```python
from build123d import *

# Parameters (mm, degrees)
BOSS_EXTRUDE1_DEPTH = 20
SKETCH2_R           = 10
BOSS_EXTRUDE2_DEPTH = 150
SKETCH3_R           = 6
CUT_EXTRUDE1_DEPTH  = 197.643421463


with BuildPart() as part:
    # Sketch1 → Boss-Extrude1 (new body)
    with BuildSketch(Plane.XY):
        with BuildLine():
            Line((-3.960100717, 69.887893103), (-2.25, 65.189429999))
            Line((-2.25, 65.189429999), (2.25, 65.189429999))
            Line((2.25, 65.189429999), (3.960100717, 69.887893103))
            ThreePointArc((3.960100717, 69.887893103), (6.100901992, 69.733628866), (8.23596739, 69.513803242))
            Line((8.23596739, 69.513803242), (9.104208278, 64.589764477))
            Line((9.104208278, 64.589764477), (13.535843167, 63.808347677))
            Line((13.535843167, 63.808347677), (16.035843167, 68.138474696))
            ThreePointArc((16.035843167, 68.138474696), (18.117333157, 67.61480784), (20.181789795, 67.027571645))
            Line((20.181789795, 67.027571645), (20.181789795, 62.027571645))
            Line((20.181789795, 62.027571645), (24.410406588, 60.488481))
            Line((24.410406588, 60.488481), (27.624344637, 64.318703216))
            ThreePointArc((27.624344637, 64.318703216), (29.583278322, 63.441545093), (31.514398729, 62.504741202))
            Line((31.514398729, 62.504741202), (30.646157841, 57.580702437))
            Line((30.646157841, 57.580702437), (34.543272158, 55.330702437))
            Line((34.543272158, 55.330702437), (38.373494373, 58.544640485))
            ThreePointArc((38.373494373, 58.544640485), (40.150350545, 57.3406431), (41.889458605, 56.082735826))
            Line((41.889458605, 56.082735826), (40.179357889, 51.384272722))
            Line((40.179357889, 51.384272722), (43.626557883, 48.491728479))
            Line((43.626557883, 48.491728479), (47.956684902, 50.991728479))
            ThreePointArc((47.956684902, 50.991728479), (49.497474683, 49.497474683), (50.991728479, 47.956684902))
            Line((50.991728479, 47.956684902), (48.491728479, 43.626557883))
            Line((48.491728479, 43.626557883), (51.384272722, 40.179357889))
            Line((51.384272722, 40.179357889), (56.082735826, 41.889458605))
            ThreePointArc((56.082735826, 41.889458605), (57.3406431, 40.150350545), (58.544640485, 38.373494373))
            Line((58.544640485, 38.373494373), (55.330702437, 34.543272158))
            Line((55.330702437, 34.543272158), (57.580702437, 30.646157841))
            Line((57.580702437, 30.646157841), (62.504741202, 31.514398729))
            ThreePointArc((62.504741202, 31.514398729), (63.441545093, 29.583278322), (64.318703216, 27.624344637))
            Line((64.318703216, 27.624344637), (60.488481, 24.410406588))
            Line((60.488481, 24.410406588), (62.027571645, 20.181789795))
            Line((62.027571645, 20.181789795), (67.027571645, 20.181789795))
            ThreePointArc((67.027571645, 20.181789795), (67.61480784, 18.117333157), (68.138474696, 16.035843167))
            Line((68.138474696, 16.035843167), (63.808347677, 13.535843167))
            Line((63.808347677, 13.535843167), (64.589764477, 9.104208278))
            Line((64.589764477, 9.104208278), (69.513803242, 8.23596739))
            ThreePointArc((69.513803242, 8.23596739), (69.733628866, 6.100901992), (69.887893103, 3.960100717))
            Line((69.887893103, 3.960100717), (65.189429999, 2.25))
            Line((65.189429999, 2.25), (65.189429999, -2.25))
            Line((65.189429999, -2.25), (69.887893103, -3.960100717))
            ThreePointArc((69.887893103, -3.960100717), (69.733628866, -6.100901992), (69.513803242, -8.23596739))
            Line((69.513803242, -8.23596739), (64.589764477, -9.104208278))
            Line((64.589764477, -9.104208278), (63.808347677, -13.535843167))
            Line((63.808347677, -13.535843167), (68.138474696, -16.035843167))
            ThreePointArc((68.138474696, -16.035843167), (67.61480784, -18.117333157), (67.027571645, -20.181789795))
            Line((67.027571645, -20.181789795), (62.027571645, -20.181789795))
            Line((62.027571645, -20.181789795), (60.488481, -24.410406588))
            Line((60.488481, -24.410406588), (64.318703216, -27.624344637))
            ThreePointArc((64.318703216, -27.624344637), (63.441545093, -29.583278322), (62.504741202, -31.514398729))
            Line((62.504741202, -31.514398729), (57.580702437, -30.646157841))
            Line((57.580702437, -30.646157841), (55.330702437, -34.543272158))
            Line((55.330702437, -34.543272158), (58.544640485, -38.373494373))
            ThreePointArc((58.544640485, -38.373494373), (57.3406431, -40.150350545), (56.082735826, -41.889458605))
            Line((56.082735826, -41.889458605), (51.384272722, -40.179357889))
            Line((51.384272722, -40.179357889), (48.491728479, -43.626557883))
            Line((48.491728479, -43.626557883), (50.991728479, -47.956684902))
            ThreePointArc((50.991728479, -47.956684902), (49.497474683, -49.497474683), (47.956684902, -50.991728479))
            Line((47.956684902, -50.991728479), (43.626557883, -48.491728479))
            Line((43.626557883, -48.491728479), (40.179357889, -51.384272722))
            Line((40.179357889, -51.384272722), (41.889458605, -56.082735826))
            ThreePointArc((41.889458605, -56.082735826), (40.150350545, -57.3406431), (38.373494373, -58.544640485))
            Line((38.373494373, -58.544640485), (34.543272158, -55.330702437))
            Line((34.543272158, -55.330702437), (30.646157841, -57.580702437))
            Line((30.646157841, -57.580702437), (31.514398729, -62.504741202))
            ThreePointArc((31.514398729, -62.504741202), (29.583278322, -63.441545093), (27.624344637, -64.318703216))
            Line((27.624344637, -64.318703216), (24.410406588, -60.488481))
            Line((24.410406588, -60.488481), (20.181789795, -62.027571645))
            Line((20.181789795, -62.027571645), (20.181789795, -67.027571645))
            ThreePointArc((20.181789795, -67.027571645), (18.117333157, -67.61480784), (16.035843167, -68.138474696))
            Line((16.035843167, -68.138474696), (13.535843167, -63.808347677))
            Line((13.535843167, -63.808347677), (9.104208278, -64.589764477))
            Line((9.104208278, -64.589764477), (8.23596739, -69.513803242))
            ThreePointArc((8.23596739, -69.513803242), (6.100901992, -69.733628866), (3.960100717, -69.887893103))
            Line((3.960100717, -69.887893103), (2.25, -65.189429999))
            Line((2.25, -65.189429999), (-2.25, -65.189429999))
            Line((-2.25, -65.189429999), (-3.960100717, -69.887893103))
            ThreePointArc((-3.960100717, -69.887893103), (-6.100901992, -69.733628866), (-8.23596739, -69.513803242))
            Line((-8.23596739, -69.513803242), (-9.104208278, -64.589764477))
            Line((-9.104208278, -64.589764477), (-13.535843167, -63.808347677))
            Line((-13.535843167, -63.808347677), (-16.035843167, -68.138474696))
            ThreePointArc((-16.035843167, -68.138474696), (-18.117333157, -67.61480784), (-20.181789795, -67.027571645))
            Line((-20.181789795, -67.027571645), (-20.181789795, -62.027571645))
            Line((-20.181789795, -62.027571645), (-24.410406588, -60.488481))
            Line((-24.410406588, -60.488481), (-27.624344637, -64.318703216))
            ThreePointArc((-27.624344637, -64.318703216), (-29.583278322, -63.441545093), (-31.514398729, -62.504741202))
            Line((-31.514398729, -62.504741202), (-30.646157841, -57.580702437))
            Line((-30.646157841, -57.580702437), (-34.543272158, -55.330702437))
            Line((-34.543272158, -55.330702437), (-38.373494373, -58.544640485))
            ThreePointArc((-38.373494373, -58.544640485), (-40.150350545, -57.3406431), (-41.889458605, -56.082735826))
            Line((-41.889458605, -56.082735826), (-40.179357889, -51.384272722))
            Line((-40.179357889, -51.384272722), (-43.626557883, -48.491728479))
            Line((-43.626557883, -48.491728479), (-47.956684902, -50.991728479))
            ThreePointArc((-47.956684902, -50.991728479), (-49.497474683, -49.497474683), (-50.991728479, -47.956684902))
            Line((-50.991728479, -47.956684902), (-48.491728479, -43.626557883))
            Line((-48.491728479, -43.626557883), (-51.384272722, -40.179357889))
            Line((-51.384272722, -40.179357889), (-56.082735826, -41.889458605))
            ThreePointArc((-56.082735826, -41.889458605), (-57.3406431, -40.150350545), (-58.544640485, -38.373494373))
            Line((-58.544640485, -38.373494373), (-55.330702437, -34.543272158))
            Line((-55.330702437, -34.543272158), (-57.580702437, -30.646157841))
            Line((-57.580702437, -30.646157841), (-62.504741202, -31.514398729))
            ThreePointArc((-62.504741202, -31.514398729), (-63.441545093, -29.583278322), (-64.318703216, -27.624344637))
            Line((-64.318703216, -27.624344637), (-60.488481, -24.410406588))
            Line((-60.488481, -24.410406588), (-62.027571645, -20.181789795))
            Line((-62.027571645, -20.181789795), (-67.027571645, -20.181789795))
            ThreePointArc((-67.027571645, -20.181789795), (-67.61480784, -18.117333157), (-68.138474696, -16.035843167))
            Line((-68.138474696, -16.035843167), (-63.808347677, -13.535843167))
            Line((-63.808347677, -13.535843167), (-64.589764477, -9.104208278))
            Line((-64.589764477, -9.104208278), (-69.513803242, -8.23596739))
            ThreePointArc((-69.513803242, -8.23596739), (-69.733628866, -6.100901992), (-69.887893103, -3.960100717))
            Line((-69.887893103, -3.960100717), (-65.189429999, -2.25))
            Line((-65.189429999, -2.25), (-65.189429999, 2.25))
            Line((-65.189429999, 2.25), (-69.887893103, 3.960100717))
            ThreePointArc((-69.887893103, 3.960100717), (-69.733628866, 6.100901992), (-69.513803242, 8.23596739))
            Line((-69.513803242, 8.23596739), (-64.589764477, 9.104208278))
            Line((-64.589764477, 9.104208278), (-63.808347677, 13.535843167))
            Line((-63.808347677, 13.535843167), (-68.138474696, 16.035843167))
            ThreePointArc((-68.138474696, 16.035843167), (-67.61480784, 18.117333157), (-67.027571645, 20.181789795))
            Line((-67.027571645, 20.181789795), (-62.027571645, 20.181789795))
            Line((-62.027571645, 20.181789795), (-60.488481, 24.410406588))
            Line((-60.488481, 24.410406588), (-64.318703216, 27.624344637))
            ThreePointArc((-64.318703216, 27.624344637), (-63.441545093, 29.583278322), (-62.504741202, 31.514398729))
            Line((-62.504741202, 31.514398729), (-57.580702437, 30.646157841))
            Line((-57.580702437, 30.646157841), (-55.330702437, 34.543272158))
            Line((-55.330702437, 34.543272158), (-58.544640485, 38.373494373))
            ThreePointArc((-58.544640485, 38.373494373), (-57.3406431, 40.150350545), (-56.082735826, 41.889458605))
            Line((-56.082735826, 41.889458605), (-51.384272722, 40.179357889))
            Line((-51.384272722, 40.179357889), (-48.491728479, 43.626557883))
            Line((-48.491728479, 43.626557883), (-50.991728479, 47.956684902))
            ThreePointArc((-50.991728479, 47.956684902), (-49.497474683, 49.497474683), (-47.956684902, 50.991728479))
            Line((-47.956684902, 50.991728479), (-43.626557883, 48.491728479))
            Line((-43.626557883, 48.491728479), (-40.179357889, 51.384272722))
            Line((-40.179357889, 51.384272722), (-41.889458605, 56.082735826))
            ThreePointArc((-41.889458605, 56.082735826), (-40.150350545, 57.3406431), (-38.373494373, 58.544640485))
            Line((-38.373494373, 58.544640485), (-34.543272158, 55.330702437))
            Line((-34.543272158, 55.330702437), (-30.646157841, 57.580702437))
            Line((-30.646157841, 57.580702437), (-31.514398729, 62.504741202))
            ThreePointArc((-31.514398729, 62.504741202), (-29.583278322, 63.441545093), (-27.624344637, 64.318703216))
            Line((-27.624344637, 64.318703216), (-24.410406588, 60.488481))
            Line((-24.410406588, 60.488481), (-20.181789795, 62.027571645))
            Line((-20.181789795, 62.027571645), (-20.181789795, 67.027571645))
            ThreePointArc((-20.181789795, 67.027571645), (-18.117333157, 67.61480784), (-16.035843167, 68.138474696))
            Line((-16.035843167, 68.138474696), (-13.535843167, 63.808347677))
            Line((-13.535843167, 63.808347677), (-9.104208278, 64.589764477))
            Line((-9.104208278, 64.589764477), (-8.23596739, 69.513803242))
            ThreePointArc((-8.23596739, 69.513803242), (-6.100901992, 69.733628866), (-3.960100717, 69.887893103))
        make_face()
    extrude(amount=BOSS_EXTRUDE1_DEPTH)

    # Sketch2 → Boss-Extrude2 (add)
    with BuildSketch(Plane.XY):
        Circle(SKETCH2_R)
    extrude(amount=-BOSS_EXTRUDE2_DEPTH)

    # Sketch3 → Cut-Extrude1 (cut, through all)
    with BuildSketch(Plane.XY.offset(20)):
        with Locations((0, 50)):
            Circle(SKETCH3_R)
    extrude(amount=-CUT_EXTRUDE1_DEPTH, mode=Mode.SUBTRACT)


solid = part.part
```
Here's how the part is built. I have some questions about the finished solid (model axes, mm). A direction names the side the tool comes from. Round coordinates to 2 decimals unless told otherwise and drop trailing zeros. Write each loop counter-clockwise with the first axis right and the second up, starting at its lowest first coordinate (ties: lowest second). Pieces come first, ordered by that corner, then holes. Notation, with made-up numbers: M 87.5,66 L 145.5,66 A20 cw 145.5,74 Z; hole C -27.75,-14.5 d9. An arc over 180 degrees is marked long. Answer as CSV lines item,"result". Start each with the question number.
1. Suppose I cut it at C-C on z = -27.5. Write out the boundary of the cut face in (x, y), then the cut area to 3 significant figures.
2. Suppose I cut it at A-A on x = 0. Write out the boundary of the cut face in (y, z), then the cut area to 3 significant figures.
3. Suppose I cut it at B-B on y = 0. Write out the boundary of the cut face in (x, z).
4. I'm going to push flat-ended pins straight in: pin 1 Ø2 at (y, z) = (-1, 6) entering from -X; pin 2 Ø5.5 at (x, z) = (64.5, 7.5) entering from +Y; pin 3 Ø1.5 at (x, z) = (-63.5, 12) entering from -Y; pin 4 Ø9.5 at (x, y) = (0, 50) entering from -Z. Where does each tip first touch, or does it pass through?
5. On a 3-axis mill with a long thin cutter (end or side, diameter ignored), from which of +Z, -Z, +X, -X, +Y, -Y can I reach the whole of each face in a straight line? I mean faces 4 (the flat face through (8.676, -67.017, 9.86)), 5 (the cylindrical face through (-2.17, -9.76, -73.95)), 6 (the flat face through (67.506, -3.093, 9.86)), 7 (the flat face through (-49.724, 45.761, 9.86)). Say none if no direction works.
6. I need wall thicknesses on probe 1 along Y at (x, z) = (0, 15); probe 2 along Z at (x, y) = (27, -48.5); probe 3 along X at (y, z) = (52.5, 6). Which ranges of each line are inside material? Lowest first, please.
7. Thinking about a two-plate mould opening in Y: for faces 1 (the flat face through (-53.701, -41.022, 9.86)), 2 (the flat face through (-11.351, 64.194, 9.86)), 3 (the flat face through (65.943, -14.768, 9.86)), which applies, released by +Y, released by -Y, zero draft, split by the parting line, or undercut?
Check result:
1,outline,"C 0,0 d20"
1,area,"314 mm2"
2,outline,"M -65.19,0 L -10,0 L -10,-150 L 10,-150 L 10,0 L 44,0 L 44,20 L -65.19,20 Z; M 56,0 L 65.19,0 L 65.19,20 L 56,20 Z"
2,area,"5,370 mm2"
3,outline,"M -65.19,0 L -10,0 L -10,-150 L 10,-150 L 10,0 L 65.19,0 L 65.19,20 L -65.19,20 Z"
4,pin 1,"stops at x = -65.19"
4,pin 2,"stops at y = 31.51"
4,pin 3,"stops at y = -31.02"
4,pin 4,"passes through"
5,face 4,"+Z, -Z, -Y"
5,face 5,"-Z"
5,face 6,"+Z, -Z, +X"
5,face 7,"+Z, -Z, -X"
6,probe 1,"y = -65.19 to 44, 56 to 65.19"
6,probe 2,"z = 0 to 20"
6,probe 3,"x = -40.59 to -5.45, 5.45 to 40.59"
7,face 1,"released by -Y"
7,face 2,"released by +Y"
7,face 3,"undercut"
